For this review, take the finished solid that the model builds, in its own axes (mm). Face numbers are marked on the shaded views. Give positions to 0.01 mm unless a question says otherwise; leave off trailing zeros. Loops run counter-clockwise (first coordinate to the right, second up) from the corner with the lowest first, then second, coordinate; pieces in that order, holes last. Notation, with made-up numbers: (34, 46) - (78, 46) arc R17 ccw to (78, 57) - close; hole circle Ø3 at (36, 29). An arc over 180 degrees is marked (long way). Answer in a Markdown table with one row per item.
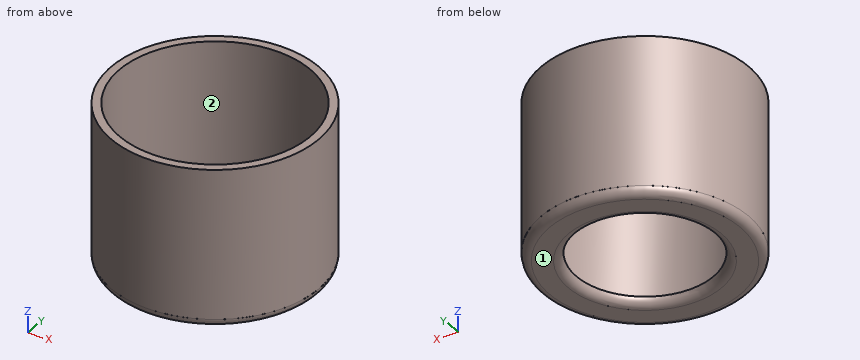
```python
from build123d import *

# Parameters (mm, degrees)
SKETCH_1_R          = 25
SKETCH_1_R_2        = 23
EXTRUDE_1_DEPTH     = 40
EXTRUDE_START       = 2
SKETCH_2_R          = 25
EXTRUDE_2_DEPTH     = 2
SKETCH_3_R          = 16.5
CUT_EXTRUDE_1_DEPTH = 2
FILLET_1_R          = 2
FILLET_2_R          = 2
FILLET_3_R          = 2
SKETCH_4_W          = 61.708706265
SKETCH_4_H          = 81.66323808
CUT_EXTRUDE_2_DEPTH = 4


with BuildPart() as part:
    # 草图1 → 凸台-拉伸1 (new body)
    with BuildSketch(Plane.XY):
        Circle(SKETCH_1_R)
        Circle(SKETCH_1_R_2, mode=Mode.SUBTRACT)
    extrude(amount=EXTRUDE_1_DEPTH)

    # 草图2 → 凸台-拉伸2 (add)
    with BuildSketch(Plane(origin=(0, 0, 0), x_dir=(-1, 0, 0), z_dir=(0, 0, -1)).offset(EXTRUDE_START)):
        Circle(SKETCH_2_R)
    extrude(amount=-EXTRUDE_2_DEPTH)

    # 草图3 → 切除-拉伸1 (cut)
    with BuildSketch(Plane(origin=(0, 0, -2), x_dir=(-1, 0, 0), z_dir=(0, 0, -1))):
        Circle(SKETCH_3_R)
    extrude(amount=-CUT_EXTRUDE_1_DEPTH, mode=Mode.SUBTRACT)

    # 圆角1
    fillet_1_edges = [part.edges().sort_by_distance(p)[0] for p in [
        (25, 0, -2),
    ]]
    fillet(fillet_1_edges, radius=FILLET_1_R - 0.0001)  # a hair under: the kernel refuses the full size

    # 圆角2
    fillet_2_edges = [part.edges().sort_by_distance(p)[0] for p in [
        (-23, 0, 0),
    ]]
    fillet(fillet_2_edges, radius=FILLET_2_R)

    # 圆角3
    fillet_3_edges = [part.edges().sort_by_distance(p)[0] for p in [
        (16.5, 0, -2),
    ]]
    fillet(fillet_3_edges, radius=FILLET_3_R - 0.0001)  # a hair under: the kernel refuses the full size

    # 草图4 → 切除-拉伸2 (cut)
    with BuildSketch(Plane.XY.offset(40)):
        with Locations((-0.068337437, -3.724390356)):
            Rectangle(SKETCH_4_W, SKETCH_4_H)
    extrude(amount=-CUT_EXTRUDE_2_DEPTH, mode=Mode.SUBTRACT)


solid = part.part
```
1. Mouldability with a two-part tool opening along X and no side actions: class the marked faces 1 and 2 as released by +X, released by -X, zero draft, split by the parting line, or undercut.
Values:
| item | result |
|---|---|
| face 1 | zero draft |
| face 2 | undercut |
2. We need section B-B, the plane z = 22. Give the boundary of the cut face in (x, y).
Values:
| item | result |
|---|---|
| outline | circle Ø50 at (0, 0); hole circle Ø46 at (0, 0) |
3. Clearance check with flat-ended pins moving along their axes: pin 1 (5 mm diameter, centred on x = 11.5, z = 8, fed in from +Y); pin 2 (5 mm diameter, centred on y = -16, z = 32, fed in from +X); pin 3 (5 mm diameter, centred on y = -14, z = 3.5, fed in from -X); pin 4 (1 mm diameter, centred on x = -8.5, y = 13.5, fed in from -Z). State where each tip first meets the part, or that it passes through.
Values:
| item | result |
|---|---|
| pin 1 | stops at y = 23.32 |
| pin 2 | stops at x = 21.04 |
| pin 3 | stops at x = -22.2 |
| pin 4 | passes through |
4. Wall thickness on line 1 (X direction, y = 0, z = 14); line 2 (Z direction, x = -20.5, y = -3): over which ranges is each line inside the solid? List them lowest first. Write a range as [from, to].
Values:
| item | result |
|---|---|
| line 1 | x = [-25, -23], [23, 25] |
| line 2 | z = [-2, 0] |
